Autodesk Inventor part; units mm, degrees
ref_plane "YZ Plane" through (0, 0, 0) normal (1, 0, 0) x (0, 1, 0)
ref_plane "XZ Plane" through (0, 0, 0) normal (0, 1, 0) x (-1, 0, 0)
ref_plane "XY Plane" through (0, 0, 0) normal (0, 0, 1) x (1, 0, 0)
sketch "Sketch1" plane through (0, 0, 0) normal (0, 0, 1) x (1, 0, 0)
  circle A0 centre (0, 0) radius 2
  dimension "Diameter" = 4
extrude "Extrusion1" add sketch "Sketch1" along normal blind 10
sketch "Sketch2" plane through (0, 0, 10) normal (0, 0, 1) x (1, 0, 0)
  circle A0 centre (0, 0) radius 2
  circle A1 centre (0, 0) radius 3.5
  dimension "Head_Diameter" = 7
extrude "Extrusion2" add sketch "Sketch2" along normal blind 4 contours A0 | A1
sketch "Sketch3" plane through (0, 0, 14) normal (0, 0, 1) x (1, 0, 0)
  circle A0 centre (0, 0) radius 3.5
  circle A1 centre (0, 0) radius 1.7321 construction
  line L0 (0, 1.7321) -> (1.5, 0.866)
  line L1 (1.5, -0.866) -> (1.5, 0.866)
  line L2 (0, 1.7321) -> (-1.5, 0.866)
  line L3 (-1.5, -0.866) -> (-1.5, 0.866)
  line L4 (-1.5, -0.866) -> (0, -1.7321)
  line L5 (1.5, -0.866) -> (0, -1.7321)
  dimension "Hex_Width" = 3
extrude "Extrusion3" cut sketch "Sketch3" against normal blind 2 contours L0 L1 L5 L4 L3 L2
thread "Thread1"
chamfer "Chamfer1" distance 0.4 angle 45 2 edges at (-3.5, 0, 14) (-2, 0, 0)
equation "\"d9\" = ThreadLength"
equation "\"d12\" = Chamfer"
equation "\"ThreadLength\" = 20"
properties part number "SCREW, SOCKET HD, P, 12_9, M4X0_7X10" material "Steel, MS"
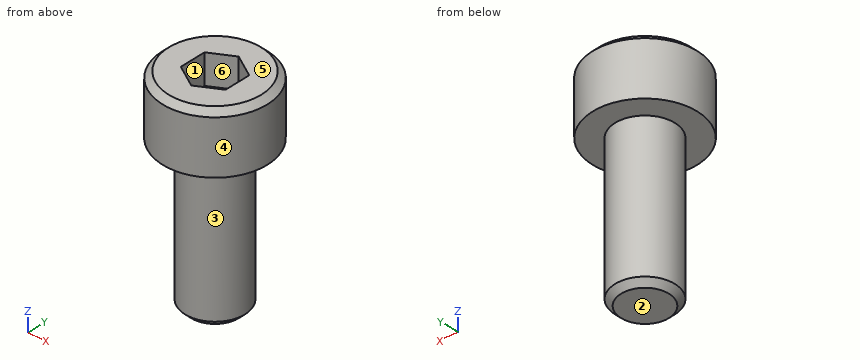
Verification items for the finished model (mm, model axes). Face numbers are marked on the shaded views. A direction names the side the tool comes from. Coordinates: 2 decimals unless noted, no trailing zeros. Order: outer loops, then holes, each group sorted by start corner. A loop starts at its lowest first (then second) coordinate and runs counter-clockwise, first axis right, second up. Notation, with made-up numbers: M -10.5,78.25 L 41.5,78.25 A17 ccw 41.5,94.25 Z; hole C -26,-34 d1. An arc over 180 degrees is marked long. One line per item, written item: value. Start each with the question number.
Item 1: Sectioned sample at B-B (z = 12.5). Enter the section's corners in (x, y), then the cut area to 3 significant figures.
Item 2: Sectioned sample at C-C (z = 11). Enter the section's corners in (x, y).
Item 3: Gauge pin test, flat ends, axial feed: pin 1 (2 mm diameter, centred on x = -2.5, z = 11.5, fed in from +Y); pin 2 (1.5 mm diameter, centred on x = -1.5, y = -2, fed in from -Z); pin 3 (0.5 mm diameter, centred on y = -0.5, z = 13, fed in from +X). Record the tip position at first contact, or that the pin passes through.
Item 4: Sectioned sample at A-A (y = 0). Enter the section's corners in (x, z).
Item 5: Mould release check, pull along X, two halves, no side actions. Record for the marked faces 4, 5 and 6: released by +X, released by -X, zero draft, split by the parting line, or undercut.
Item 6: Scan lines: probe 1 along Z at (x, y) = (-1.5, -1.75); probe 2 along Z at (x, y) = (0.75, -0.75); probe 3 along Y at (x, z) = (0.5, 12.25). Record each from-to range of solid material in increasing order.
Item 7: Access from +Z, -Z, +X, -X, +Y, -Y to the whole of each face (thin tool, end or side, straight path). Record for the marked faces 1, 2 and 3.
Item 8: Sectioned sample at D-D (z = 4.5). Enter the section's corners in (x, y), then the cut area to 3 significant figures.
Conclusion:
1. outline: C 0,0 d7; hole M -1.5,-0.87 L 0,-1.73 L 1.5,-0.87 L 1.5,0.87 L 0,1.73 L -1.5,0.87 Z
1. area: 30.7 mm^2
2. outline: C 0,0 d7
3. pin 1: stops at y = 3.16
3. pin 2: stops at z = 0.15
3. pin 3: stops at x = 3.49
4. outline: M -3.5,10 L -2,10 L -2,0.4 L -1.6,0 L 1.6,0 L 2,0.4 L 2,10 L 3.5,10 L 3.5,13.6 L 3.1,14 L 1.5,14 L 1.5,12 L -1.5,12 L -1.5,14 L -3.1,14 L -3.5,13.6 Z
5. face 4: split by the parting line
5. face 5: zero draft
5. face 6: undercut
6. probe 1: z = 10 to 14
6. probe 2: z = 0 to 12
6. probe 3: y = -3.46 to -1.44, 1.44 to 3.46
7. face 1: +Z
7. face 2: -Z, +X, -X, +Y, -Y
7. face 3: -Z
8. outline: C 0,0 d4
8. area: 12.6 mm^2
